Source: CAD feature listing. Evaluate the final solid. Frame: model axes, mm. Face numbers are marked on the shaded views. A direction names the side the tool comes from. Round coordinates to 2 decimals unless told otherwise and drop trailing zeros. Loops run counter-clockwise (first coordinate to the right, second up) from the corner with the lowest first, then second, coordinate; pieces in that order, holes last.
(1) Set-up query: the marked faces 1, 2 and 3. Return all of +Z, -Z, +X, -X, +Y, -Y with unobstructed straight access to the full face (end or side cutting, diameter ignored); none if empty.
(2) First-contact query: pin 1 Ø12.5 at (x, z) = (-33.5, 8) entering from +Y; pin 2 Ø9 at (x, z) = (38.1, 12.7) entering from +Y; pin 3 Ø12.5 at (y, z) = (24, 15) entering from +X; pin 4 Ø12 at (x, y) = (-11.5, 27) entering from -Z. Flat tips, straight axial feed; report the tip coordinate or a pass-through.
(3) Section D-D, the plane z = 12.7. Count the separate pieces of the cut face and the enclosed holes in it, plus the area to 3 significant figures.
(4) Material intervals for probe 1 along X at (y, z) = (4, 12.7); probe 2 along Z at (x, y) = (38, 5); probe 3 along Z at (x, y) = (38, 10), sorted ascending.
(5) Mould query, pull axis Z, two halves, no side actions, for the marked faces 4, 5 and 6. Classes: pulls with the +Z half, pulls with the -Z half, needs draft (parallel to the pull), parting line crosses it, or undercut.
(6) Section C-C, the plane y = 26. Return the cut outline in (x, z), plus the area to 3 significant figures.
(7) Section A-A, the plane x = -38.1. Return the cut outline in (y, z), plus the area to 3 significant figures.
(8) Section B-B, the plane y = 39. Return the cut outline in (x, z).
```python
from build123d import *

# Parameters (mm, degrees)
BOSS_EXTRUDE1_DEPTH                              = 25.4
CBORE_FOR_1_4_SOCKET_HEAD_CAP_SCREW1_D           = 6.7564
CBORE_FOR_1_4_SOCKET_HEAD_CAP_SCREW1_CBORE_D     = 11.1125
CBORE_FOR_1_4_SOCKET_HEAD_CAP_SCREW1_CBORE_DEPTH = 6.35
SKETCH6_R                                        = 7.9375
CUT_EXTRUDE2_DEPTH                               = 93.898049386


with BuildPart() as part:
    # Sketch1 → Boss-Extrude1 (new body)
    with BuildSketch(Plane.XY):
        Polygon((25.4, 12.7), (50.8, 12.7), (50.8, 0), (-50.8, 0), (-50.8, 12.7), (-25.4, 12.7), (-25.4, 50.8), (25.4, 50.8), align=None)
    extrude(amount=BOSS_EXTRUDE1_DEPTH)

    # CBORE for 1/4 Socket Head Cap Screw1 (through all)
    with Locations(Plane(origin=(0, 12.7, 0), x_dir=(1, 0, 0), z_dir=(0, 1, 0))):
        with Locations((-38.1, -12.7), (38.1, -12.7)):
            CounterBoreHole(CBORE_FOR_1_4_SOCKET_HEAD_CAP_SCREW1_D / 2, CBORE_FOR_1_4_SOCKET_HEAD_CAP_SCREW1_CBORE_D / 2, CBORE_FOR_1_4_SOCKET_HEAD_CAP_SCREW1_CBORE_DEPTH)

    # Sketch6 → Cut-Extrude2 (cut, through all)
    with BuildSketch(Plane(origin=(-10.442463605, 32.464422505, 61.850379973), x_dir=(-0.9762276715802475, 0.026604535934103283, -0.21510865140374857), z_dir=(0.21650558359918726, 0.07280416213947143, -0.9735629852482811))):
        Circle(SKETCH6_R)
        with BuildLine():
            Line((-6.795136978, 42.915355356), (-7.934675442, 0.211735396))
            ThreePointArc((-7.934675442, 0.211735396), (0.105877117, 7.936793829), (7.9375, 0))
            ThreePointArc((7.9375, 0), (7.936793829, -0.105877117), (7.934675442, -0.211735396))
            Line((7.934675442, -0.211735396), (9.074213906, 42.491884564))
            Line((9.074213906, 42.491884564), (-6.795136978, 42.915355356))
        make_face()
    extrude(amount=CUT_EXTRUDE2_DEPTH, mode=Mode.SUBTRACT)


solid = part.part
```
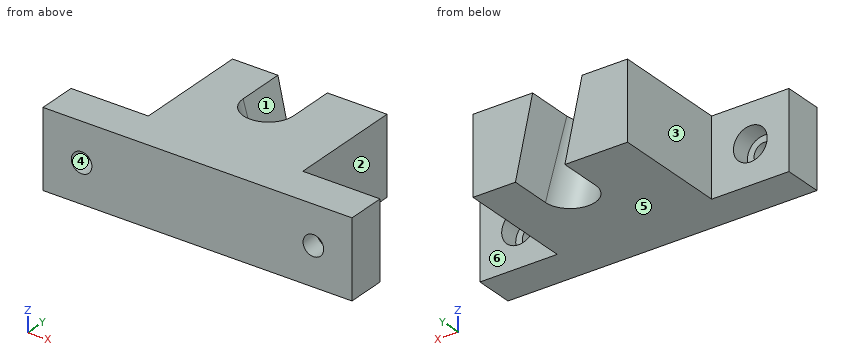
Output values:
1. face 1: +Z, +Y
1. face 2: +Z, -Z, +X, +Y
1. face 3: +Z, -Z, -X, +Y
2. pin 1: stops at y = 12.7
2. pin 2: stops at y = 6.35
2. pin 3: stops at x = 25.4
2. pin 4: stops at z = 0
3. separate pieces: 3
3. enclosed holes: 0
3. area: 2,660 mm2
4. probe 1: x = -50.8 to -41.48, -34.72 to 34.72, 41.48 to 50.8
4. probe 2: z = 0 to 9.32, 16.08 to 25.4
4. probe 3: z = 0 to 7.14, 18.26 to 25.4
5. face 4: undercut
5. face 5: pulls with the -Z half
5. face 6: needs draft
6. outline: (-25.4, 0) - (25.4, 0) - (25.4, 25.4) - (-25.4, 25.4) - close
6. area: 1,290 mm2
7. outline: (0, 0) - (12.7, 0) - (12.7, 7.14) - (6.35, 7.14) - (6.35, 9.32) - (0, 9.32) - close; (0, 16.08) - (6.35, 16.08) - (6.35, 18.26) - (12.7, 18.26) - (12.7, 25.4) - (0, 25.4) - close
7. area: 209 mm2
8. outline: (-25.4, 0) - (-4.82, 0) - (-10.47, 25.4) - (-25.4, 25.4) - close; (5.79, 25.4) - (11.44, 0) - (25.4, 0) - (25.4, 25.4) - close
